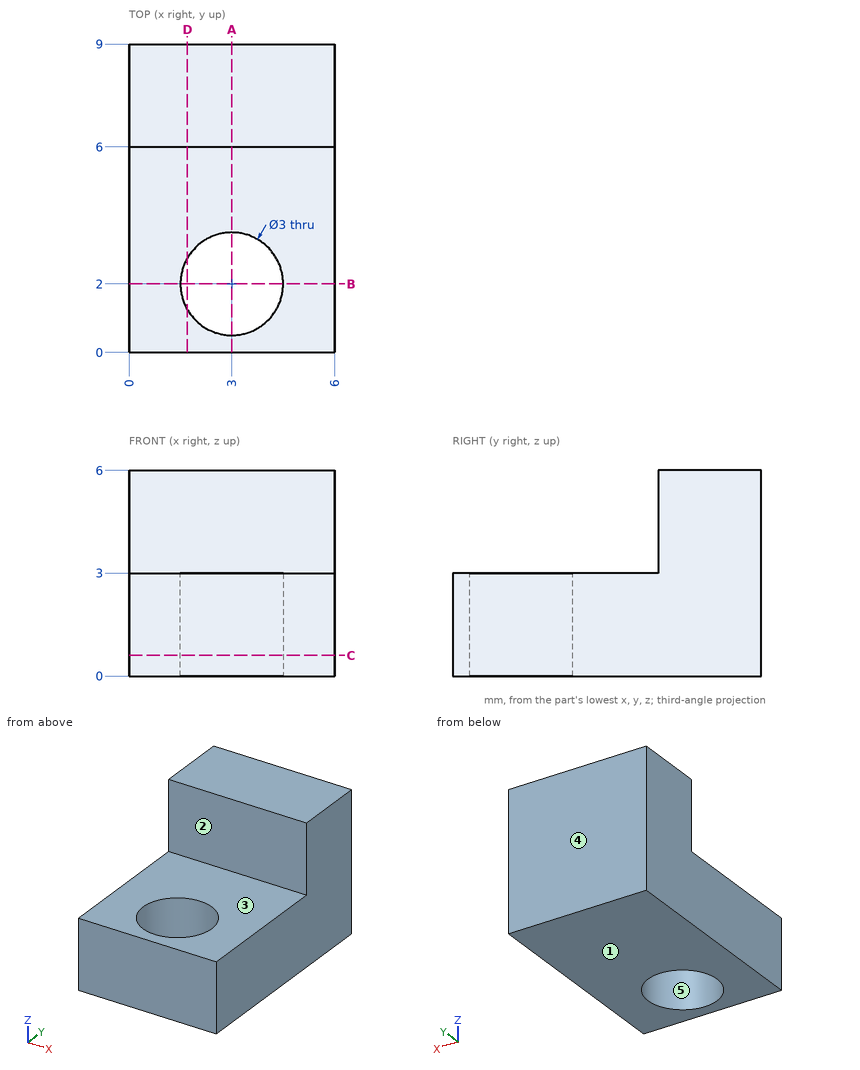
Source: three-view drawing plus pictorial views. Frame: mm from the lowest corner of the part. A direction names the side the tool comes from. Round coordinates to 2 decimals unless told otherwise and drop trailing zeros. Loops run counter-clockwise (first coordinate to the right, second up) from the corner with the lowest first, then second, coordinate; pieces in that order, holes last.
1. Ray query, L1, parallel to Y at x = 3, z = 1.7; L2, parallel to Z at x = 1.7, y = 3.75; L3, parallel to X at y = 2.5, z = 2.3. Return the intervals inside material, ascending.
2. Section query A-A on x = 3. Output: boundary loops of the cut face in (y, z), and give its area (3 significant figures).
3. Section query C-C on z = 0.6. Output: boundary loops of the cut face in (x, y), and give its area (3 significant figures).
4. Section query D-D on x = 1.7. Output: boundary loops of the cut face in (y, z), and give its area (3 significant figures).
5. Contact query for a flat-ended pin moving along its axis: pin 1 (3 mm diameter, centred on x = 2.5, y = 3.5, fed in from +Z). Output: stop coordinate, or through.
6. Section query B-B on y = 2. Output: boundary loops of the cut face in (x, z).
7. Access query for the marked faces 1 and 2. Directions: +Z, -Z, +X, -X, +Y, -Y. A direction counts if a zero-diameter tool reaches every point of the face in a straight line with its end or side. Return the directions, or none.
8. Mould query, pull axis Y, two halves, no side actions, for the marked faces 3, 4 and 5. Classes: released by +Y, released by -Y, zero draft, split by the parting line, or undercut.
Answers below:
1. L1: y = 0 to 0.5, 3.5 to 9
1. L2: z = 0 to 3
1. L3: x = 0 to 1.59, 4.41 to 6
2. outline: (0, 0) - (0.5, 0) - (0.5, 3) - (0, 3) - close; (3.5, 0) - (9, 0) - (9, 6) - (6, 6) - (6, 3) - (3.5, 3) - close
2. area: 27.0 mm2
3. outline: (0, 0) - (6, 0) - (6, 9) - (0, 9) - close; hole circle Ø3 at (3, 2)
3. area: 46.9 mm2
4. outline: (0, 0) - (1.25, 0) - (1.25, 3) - (0, 3) - close; (2.75, 0) - (9, 0) - (9, 6) - (6, 6) - (6, 3) - (2.75, 3) - close
4. area: 31.5 mm2
5. pin 1: stops at z = 3
6. outline: (0, 0) - (1.5, 0) - (1.5, 3) - (0, 3) - close; (4.5, 0) - (6, 0) - (6, 3) - (4.5, 3) - close
7. face 1: -Z, +X, -X, +Y, -Y
7. face 2: +Z, +X, -X, -Y
8. face 3: zero draft
8. face 4: released by +Y
8. face 5: undercut
